Could you check a few things on this model? Use its own coordinates, in mm. A direction names the side the tool comes from. Give positions to 0.01 mm unless a question says otherwise; leave off trailing zeros. Write each loop counter-clockwise with the first axis right and the second up, starting at its lowest first coordinate (ties: lowest second). Pieces come first, ordered by that corner, then holes. Notation, with made-up numbers: (51, 58) - (94, 58) arc R21 ccw to (94, 93) - close; hole circle Ø5 at (18.5, 43.25). An arc over 180 degrees is marked (long way). Use one line per item in the form item = value.
Autodesk Inventor part; units mm, degrees
ref_plane "YZ Plane" through (0, 0, 0) normal (1, 0, 0) x (0, 1, 0)
ref_plane "XZ Plane" through (0, 0, 0) normal (0, 1, 0) x (-1, 0, 0)
ref_plane "XY Plane" through (0, 0, 0) normal (0, 0, 1) x (1, 0, 0)
sketch "Sketch1" plane through (0, 0, 0) normal (0, 1, 0) x (-1, 0, 0)
  circle A0 centre (0, 0) radius 57.15
  dimension "d0" = 114.3
extrude "Extrusion1" add sketch "Sketch1" along normal blind 3.175
sketch "Sketch2" plane through (0, 3.175, 0) normal (0, 1, 0) x (1, 0, 0)
  circle A0 centre (0, 0) radius 50.8
  circle A1 centre (0, 0) radius 49.2125
  dimension "d3" = 101.6
  dimension "d4" = 98.425
extrude "Extrusion2" add sketch "Sketch2" along normal blind 45.72
sketch "Sketch3" plane through (0, 3.175, 0) normal (0, 1, 0) x (1, 0, 0)
  circle A0 centre (0, 0) radius 49.2125
extrude "Extrusion3" add sketch "Sketch3" along normal blind 4.7625
sketch "Sketch4" plane through (0, 0, 0) normal (0, -1, 0) x (1, 0, 0)
  line L0 (3.175, 3.175) -> (34.925, 3.175)
  line L1 (34.925, 3.175) -> (34.925, -3.175)
  line L2 (34.925, -3.175) -> (3.175, -3.175)
  line L3 (3.175, -3.175) -> (3.175, -34.925)
  line L4 (3.175, -34.925) -> (-3.175, -34.925)
  line L5 (-3.175, -34.925) -> (-3.175, -3.175)
  line L6 (-3.175, -3.175) -> (-34.925, -3.175)
  line L7 (-34.925, -3.175) -> (-34.925, 3.175)
  line L8 (-34.925, 3.175) -> (-3.175, 3.175)
  line L9 (-3.175, 3.175) -> (-3.175, 34.925)
  line L10 (-3.175, 34.925) -> (3.175, 34.925)
  line L11 (3.175, 34.925) -> (3.175, 3.175)
  point P0 (0, 0)
  dimension "d9" = 31.75
  dimension "d10" = 6.35
  dimension "d11" = 31.75
  dimension "d12" = 6.35
  dimension "d13" = 31.75
  dimension "d14" = 31.75
extrude "Extrusion4" cut sketch "Sketch4" against normal blind 6.35
properties part number "Base Plug"
1. Imagine slicing it at C-C, the plane y = 22. List the corners of the cut face in (x, z) for me (1 decimal).
Response values:
outline = circle Ø101.6 at (0, 0); hole circle Ø98.4 at (0, 0)
2. Imagine slicing it at D-D, the plane z = -38.5. List the corners of the cut face in (x, y) for me (1 decimal), and give its area (3 significant figures).
Response values:
outline = (-42.2, 0) - (42.2, 0) - (42.2, 3.2) - (33.1, 3.2) - (33.1, 48.9) - (30.7, 48.9) - (30.7, 7.9) - (-30.7, 7.9) - (-30.7, 48.9) - (-33.1, 48.9) - (-33.1, 3.2) - (-42.2, 3.2) - close
area = 788 mm²
3. For pin 1 (1.9 mm diameter, centred on x = -1, y = 2, fed in from -Z); pin 2 (1 mm diameter, centred on x = 0, y = 14.5, fed in from +Z); pin 3 (3 mm diameter, centred on y = 2, z = -21.5, fed in from +X), each with a flat end and sliding along its axis, tell me the tip position at first contact or that it passes through.
Response values:
pin_1 = -57.15
pin_2 = 50.8
pin_3 = 53.54
4. If we mould it in two halves opening along Z, with no side actions, what happens to faces 4 (the face through (-12, 0, -12)), 5 (the face through (57.095, 1.565, -2.513)), 6 (the face through (-34.925, 3, 0))? For each: pulls with the +Z half, pulls with the -Z half, needs draft (parallel to the pull), parting line crosses it, or undercut.
Response values:
face_4 = needs draft
face_5 = parting line crosses it
face_6 = undercut
5. If I drill on line 1 (X direction, y = 17, z = 0); line 2 (Y direction, x = 32.5, z = -19), over which ranges is the centre line in solid material (lowest first)? Write a range as from..to.
Response values:
line_1 = -50.8..-49.21, 49.21..50.8
line_2 = 0..7.94
6. Which directions (+Z, -Z, +X, -X, +Y, -Y) give clear straight access to the entire face, cutting with the end or side of a thin tool? Please do faces 1 (the face through (-19, 3, -3.175)), 2 (the face through (46.94, 28.13, 14.78)), 3 (the face through (-27, 48.895, -42)).
Response values:
face_1 = -Y
face_2 = +Y
face_3 = +Z, -Z, +X, -X, +Y
